Source: CAD feature listing. Evaluate the final solid. Frame: model axes, mm. Face numbers are marked on the shaded views. Coordinates: 2 decimals unless noted, no trailing zeros. Order: outer loops, then holes, each group sorted by start corner. A loop starts at its lowest first (then second) coordinate and runs counter-clockwise, first axis right, second up.
Item 1: Section B-B on z = 0. Return the cut outline in (x, y), then the cut area to 3 significant figures.
Item 2: Mould query, pull axis X, two halves, no side actions, for the marked faces 1, 2 and 3. Classes: released by +X, released by -X, zero draft, split by the parting line, or undercut.
Item 3: Contact query for flat-ended pins moving along their axis: P1, Ø8, axis at x = 5.5, y = 80.5, coming from the +Z side; P2, Ø1, axis at x = -6.5, z = -0.5, coming from the +Y side; P3, Ø3, axis at x = 3.5, y = 42, coming from the -Z side. Output: stop coordinate, or through.
Item 4: Section A-A on x = 0. Return the cut outline in (y, z).
Item 5: Section C-C on y = 96. Return the cut outline in (x, z), then the cut area to 3 significant figures.
Item 6: Ray query, line 1 (Y direction, x = -6.25, z = -2); line 2 (X direction, y = 93.5, z = 0.75); line 3 (X direction, y = 83.5, z = 0.25). Return the intervals inside material, ascending.
Item 7: Section D-D on x = -5. Return the cut outline in (y, z).
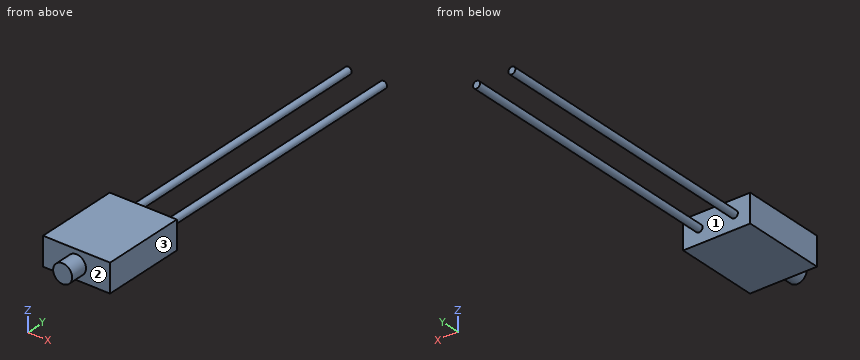
from build123d import *

# Parameters (mm, degrees)
SKETCH_1_W      = 19
SKETCH_1_H      = 8
EXTRUDE_1_DEPTH = 24
SKETCH_2_R      = 1
EXTRUDE_2_DEPTH = 80
SKETCH_3_R      = 2.686102283
EXTRUDE_3_DEPTH = 5


with BuildPart() as part:
    # 草图1 → 凸台-拉伸1 (new body)
    with BuildSketch(Plane(origin=(0, 0, 0), x_dir=(1, 0, 0), z_dir=(0, 1, 0))):
        Rectangle(SKETCH_1_W, SKETCH_1_H)
    extrude(amount=EXTRUDE_1_DEPTH)

    # 草图2 → 凸台-拉伸2 (add)
    with BuildSketch(Plane(origin=(0, 24, 0), x_dir=(1, 0, 0), z_dir=(0, 1, 0))):
        with Locations((5, 0)):
            Circle(SKETCH_2_R)
        with Locations((-5, 0)):
            Circle(SKETCH_2_R)
    extrude(amount=EXTRUDE_2_DEPTH)

    # 草图3 → 凸台-拉伸3 (add)
    with BuildSketch(Plane.XZ):
        Circle(SKETCH_3_R)
    extrude(amount=EXTRUDE_3_DEPTH)


solid = part.part
Answer list:
1. outline: (-9.5, 0) - (-2.69, 0) - (-2.69, -5) - (2.69, -5) - (2.69, 0) - (9.5, 0) - (9.5, 24) - (6, 24) - (6, 104) - (4, 104) - (4, 24) - (-4, 24) - (-4, 104) - (-6, 104) - (-6, 24) - (-9.5, 24) - close
1. area: 803 mm2
2. face 1: undercut
2. face 2: zero draft
2. face 3: released by +X
3. P1: stops at z = 1
3. P2: stops at y = 24
3. P3: stops at z = -1
4. outline: (-5, -2.69) - (0, -2.69) - (0, -4) - (24, -4) - (24, 4) - (0, 4) - (0, 2.69) - (-5, 2.69) - close
5. outline: circle Ø2 at (-5, 0); circle Ø2 at (5, 0)
5. area: 6.28 mm2
6. line 1: y = 0 to 24
6. line 2: x = -5.66 to -4.34, 4.34 to 5.66
6. line 3: x = -5.97 to -4.03, 4.03 to 5.97
7. outline: (0, -4) - (24, -4) - (24, -1) - (104, -1) - (104, 1) - (24, 1) - (24, 4) - (0, 4) - close
